Autodesk Inventor part; units mm, degrees
ref_plane "YZ Plane" through (0, 0, 0) normal (1, 0, 0) x (0, 1, 0)
ref_plane "XZ Plane" through (0, 0, 0) normal (0, 1, 0) x (-1, 0, 0)
ref_plane "XY Plane" through (0, 0, 0) normal (0, 0, 1) x (1, 0, 0)
sketch "_____1" plane through (0, 0, 0) normal (0, 0, 1) x (1, 0, 0)
  arc A0 (0, 8.52) -> (0, -8.52) centre (0, 0) ccw
  line L0 (0, -8.52) -> (769.5, -8.52)
  arc A1 (769.5, -8.52) -> (769.5, 8.52) centre (769.5, 0) ccw
  line L1 (769.5, 8.52) -> (0, 8.52)
  arc A2 (0, 7.26) -> (0, -7.26) centre (0, 0) ccw
  line L2 (0, -7.26) -> (769.5, -7.26)
  arc A3 (769.5, -7.26) -> (769.5, 7.26) centre (769.5, 0) ccw
  line L3 (769.5, 7.26) -> (0, 7.26)
extrude "Extrusion1" add sketch "_____1" along normal mid plane 15
sketch "_____2" plane through (0, 0, 0) normal (0, 0, 1) x (1, 0, 0)
  line L0 (377.25, 8.52) -> (377.25, 7.26)
  line L1 (377.25, 7.26) -> (377.6077, 7.26)
  arc A0 (377.8552, 7.0453) -> (377.6077, 7.26) centre (377.6077, 7.01) ccw
  arc A1 (377.8552, 7.0453) -> (377.9317, 6.7401) centre (379.36, 7.26) ccw
  arc A2 (377.9317, 6.7401) -> (379.5683, 6.7401) centre (378.75, 6.97) ccw
  arc A3 (379.5683, 6.7401) -> (379.6448, 7.0453) centre (378.14, 7.26) ccw
  arc A4 (379.8923, 7.26) -> (379.6448, 7.0453) centre (379.8923, 7.01) ccw
  line L2 (379.8923, 7.26) -> (380.6077, 7.26)
  arc A5 (380.8552, 7.0453) -> (380.6077, 7.26) centre (380.6077, 7.01) ccw
  arc A6 (380.8552, 7.0453) -> (380.9317, 6.7401) centre (382.36, 7.26) ccw
  arc A7 (380.9317, 6.7401) -> (382.5683, 6.7401) centre (381.75, 6.97) ccw
  arc A8 (382.5683, 6.7401) -> (382.6448, 7.0453) centre (381.14, 7.26) ccw
  arc A9 (382.8923, 7.26) -> (382.6448, 7.0453) centre (382.8923, 7.01) ccw
  line L3 (382.8923, 7.26) -> (383.6077, 7.26)
  arc A10 (383.8552, 7.0453) -> (383.6077, 7.26) centre (383.6077, 7.01) ccw
  arc A11 (383.8552, 7.0453) -> (383.9317, 6.7401) centre (385.36, 7.26) ccw
  arc A12 (383.9317, 6.7401) -> (385.5683, 6.7401) centre (384.75, 6.97) ccw
  arc A13 (385.5683, 6.7401) -> (385.6448, 7.0453) centre (384.14, 7.26) ccw
  arc A14 (385.8923, 7.26) -> (385.6448, 7.0453) centre (385.8923, 7.01) ccw
  line L4 (385.8923, 7.26) -> (386.6077, 7.26)
  arc A15 (386.8552, 7.0453) -> (386.6077, 7.26) centre (386.6077, 7.01) ccw
  arc A16 (386.8552, 7.0453) -> (386.9317, 6.7401) centre (388.36, 7.26) ccw
  arc A17 (386.9317, 6.7401) -> (388.5683, 6.7401) centre (387.75, 6.97) ccw
  arc A18 (388.5683, 6.7401) -> (388.6448, 7.0453) centre (387.14, 7.26) ccw
  arc A19 (388.8923, 7.26) -> (388.6448, 7.0453) centre (388.8923, 7.01) ccw
  line L5 (388.8923, 7.26) -> (389.6077, 7.26)
  arc A20 (389.8552, 7.0453) -> (389.6077, 7.26) centre (389.6077, 7.01) ccw
  arc A21 (389.8552, 7.0453) -> (389.9317, 6.7401) centre (391.36, 7.26) ccw
  arc A22 (389.9317, 6.7401) -> (391.5683, 6.7401) centre (390.75, 6.97) ccw
  arc A23 (391.5683, 6.7401) -> (391.6448, 7.0453) centre (390.14, 7.26) ccw
  arc A24 (391.8923, 7.26) -> (391.6448, 7.0453) centre (391.8923, 7.01) ccw
  line L6 (391.8923, 7.26) -> (392.25, 7.26)
  line L7 (392.25, 7.26) -> (392.25, 8.52)
  line L8 (392.25, 8.52) -> (377.25, 8.52)
extrude "Extrusion2" add sketch "_____2" along normal mid plane 15
properties part number "GBN1587MR3-150_info-1-16-16"
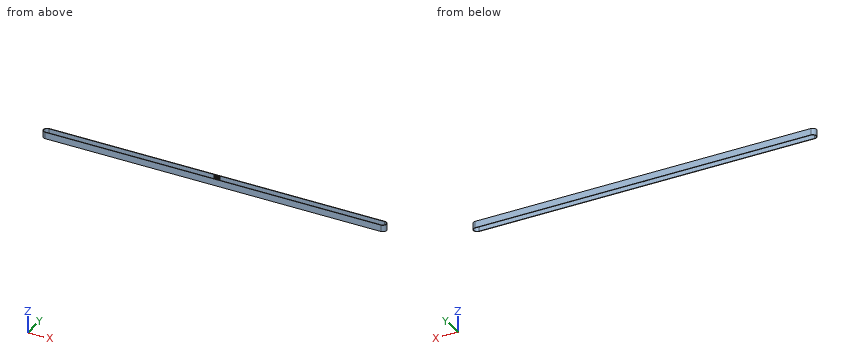
The model under review builds one solid part; all positions refer to its coordinate system, in mm. Give positions to 0.01 mm unless a question says otherwise; leave off trailing zeros. Order: outer loops, then holes, each group sorted by start corner. A loop starts at its lowest first (then second) coordinate and runs counter-clockwise, first axis right, second up. Notation, with made-up numbers: (29, -34.5) -> (33, -34.5) arc R25 ccw to (33, -7.5) -> close; hole circle Ø8 at (65, -20). An arc over 180 degrees is marked (long way). Write item = value, one per line. Start each with the question number.
(1) For pin 1 Ø1 at (y, z) = (-6.5, 3) entering from -X; pin 2 Ø1.5 at (y, z) = (-2, 5) entering from -X; pin 3 Ø1.5 at (y, z) = (-4, -6) entering from +X, all flat-tipped, find the tip position at first contact; note any pin that passes through.
(2) For L1, parallel to X at y = -1, z = -4.5; L2, parallel to Y at x = 585.5, z = -1; L3, parallel to X at y = 1.25, z = 5.75, list the stretches that pass through material, from the lowest coordinate up. Write a range as from..to.
(3) Take a section at A-A (x = 315.5). Write out the cut boundary in (y, z).
(4) Take a section at B-B (y = 0). Write out the cut boundary in (x, z), plus the area to 3 significant figures.
Returned:
q1.pin_1 = -6.05
q1.pin_2 = -8.43
q1.pin_3 = 777.38
q2.L1 = -8.46..-7.19, 776.69..777.96
q2.L2 = -8.52..-7.26, 7.26..8.52
q2.L3 = -8.43..-7.15, 776.65..777.93
q3.outline = (-8.52, -7.5) -> (-7.26, -7.5) -> (-7.26, 7.5) -> (-8.52, 7.5) -> close; (7.26, -7.5) -> (8.52, -7.5) -> (8.52, 7.5) -> (7.26, 7.5) -> close
q4.outline = (-8.52, -7.5) -> (-7.26, -7.5) -> (-7.26, 7.5) -> (-8.52, 7.5) -> close; (776.76, -7.5) -> (778.02, -7.5) -> (778.02, 7.5) -> (776.76, 7.5) -> close
q4.area = 37.8 mm²
